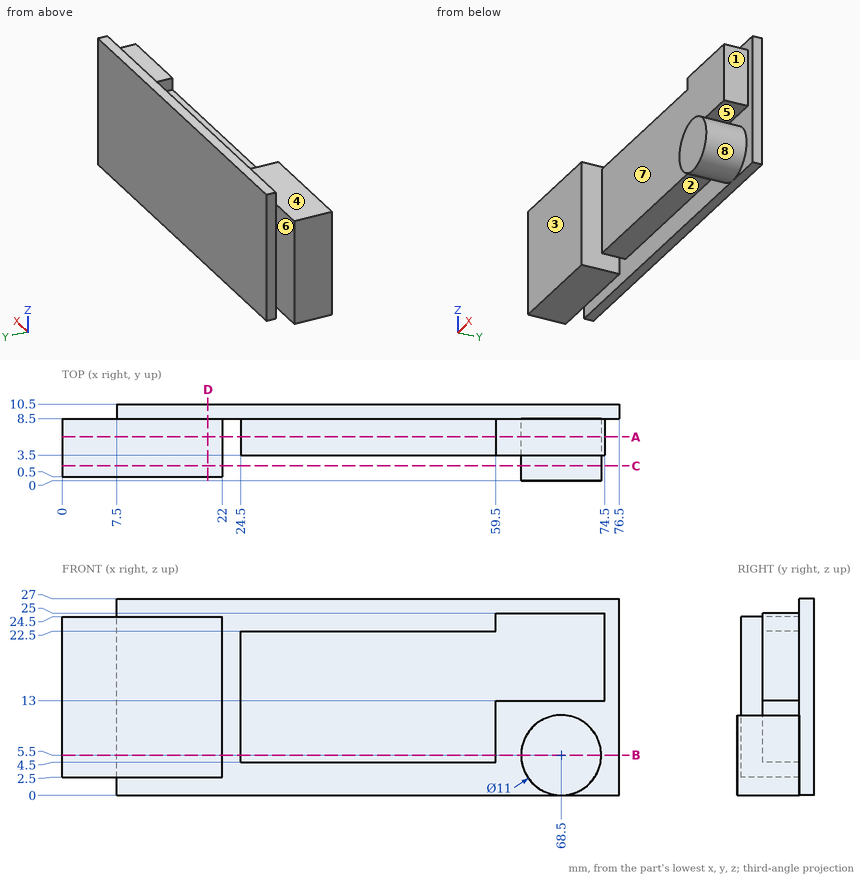
Answer from the drawing. Dimensions are ordinates in mm from the lowest x, y and z of the part. A direction names the side the tool comes from. Coordinates: 2 decimals unless noted, no trailing zeros. Write each loop counter-clockwise with the first axis right and the second up, starting at its lowest first coordinate (ties: lowest second). Pieces come first, ordered by that corner, then holes. Notation, with made-up numbers: M 38,59 L 72,59 A20 ccw 72,80 Z; hole C 66,39 d11. An arc over 180 degrees is marked long. Use one line per item in the form item = value. Start each with the question number.
1. A tool of negligible diameter and unlimited length cuts with its end or side. For the marked faces 4, 5, 6, 7 and 8, from which of +Z, -Z, +X, -X, +Y, -Y can it reach the whole face along a straight path? Write none if from no direction.
2. The mould has two halves that part along X. Classify the marked faces 1, 2 and 3: released by +X, released by -X, zero draft, split by the parting line, or undercut.
3. Each of these flat-tipped pins is pushed along its axis until it touches: P1, Ø1.5, axis at y = 6.5, z = 19, coming from the +X side; P2, Ø11, axis at x = 8, z = 8.5, coming from the -Y side; P3, Ø2.5, axis at x = 69.5, y = 5.5, coming from the +Z side. Where does it stop, or does it pass through?
4. The part is cut by section B-B (z = 5.5). Give the vertices of the cut face in (x, y), plus the area to 4 significant figures.
5. The part is cut by section A-A (y = 6). Give the vertices of the cut face in (x, z).
6. The part is cut by section C-C (y = 2). Give the vertices of the cut face in (x, z).
7. Straight lines are drawn through the part: probe 1 along X at (y, z) = (5.25, 21.25); probe 2 along Z at (x, y) = (15.5, 2.5); probe 3 along X at (y, z) = (9.75, 22.5). For each, find the intervals that lie inside material, in ascending order. Write a range as from..to.
8. The part is cut by section D-D (x = 20). Give the vertices of the cut face in (y, z), plus the area to 3 significant figures.
Evaluation:
q1.face_4 = +Z, -X, -Y
q1.face_5 = +X, -Y
q1.face_6 = +Z, -Z, -X, +Y
q1.face_7 = +Z, -Y
q1.face_8 = -Y
q2.face_1 = released by +X
q2.face_2 = undercut
q2.face_3 = zero draft
q3.P1 = 74.5
q3.P2 = 0.5
q3.P3 = 25
q4.outline = M 0,0.5 L 22,0.5 L 22,8.5 L 24.5,8.5 L 24.5,3.5 L 59.5,3.5 L 59.5,8.5 L 63,8.5 L 63,0 L 74,0 L 74,8.5 L 76.5,8.5 L 76.5,10.5 L 7.5,10.5 L 7.5,8.5 L 0,8.5 Z
q4.area = 582.5 mm^2
q5.outline = M 0,2.5 L 22,2.5 L 22,24.5 L 0,24.5 Z; M 24.5,4.5 L 59.5,4.5 L 59.5,13 L 74.5,13 L 74.5,25 L 59.5,25 L 59.5,22.5 L 24.5,22.5 Z; C 68.5,5.5 d11
q6.outline = M 0,2.5 L 22,2.5 L 22,24.5 L 0,24.5 Z; C 68.5,5.5 d11
q7.probe_1 = 0..22, 24.5..74.5
q7.probe_2 = 2.5..24.5
q7.probe_3 = 7.5..76.5
q8.outline = M 0.5,2.5 L 8.5,2.5 L 8.5,0 L 10.5,0 L 10.5,27 L 8.5,27 L 8.5,24.5 L 0.5,24.5 Z
q8.area = 230 mm^2
